Verification items for the finished model (mm, model axes). A direction names the side the tool comes from. Coordinates: 2 decimals unless noted, no trailing zeros. Order: outer loops, then holes, each group sorted by start corner. A loop starts at its lowest first (then second) coordinate and runs counter-clockwise, first axis right, second up. Notation, with made-up numbers: (-14, 42) -> (-1, 42) arc R20 ccw to (-1, 59) -> close; hole circle Ø3 at (30, 79). An arc over 180 degrees is marked (long way). Answer as CSV lines item,"result".
```python
from build123d import *

# Parameters (mm, degrees)
BOSS_EXTRUDE1_DEPTH  = 3.5
SKETCH3_R            = 4
CUT_EXTRUDE1_DEPTH   = 12.35
M5_CLEARANCE_HOLE1_D = 5.3


with BuildPart() as part:
    # Sketch1 → Boss-Extrude1 (new body)
    with BuildSketch(Plane(origin=(0, 0, 0), x_dir=(1, 0, 0), z_dir=(0, 1, 0))):
        with BuildLine():
            Line((-23.15, 0), (0, 0))
            Line((0, 0), (0, 13.4))
            ThreePointArc((0, 13.4), (-3.214400781, 13.008751962), (-6.24109589, 11.857854869))
            Line((-6.24109589, 11.857854869), (-20.532191781, 4.336081258))
            ThreePointArc((-20.532191781, 4.336081258), (-22.44480272, 2.532514588), (-23.15, 0))
        make_face()
    extrude(amount=BOSS_EXTRUDE1_DEPTH)

    # Mirror3: part across plane


with BuildPart() as part_1:
    add(part.part)
    add(part.part.mirror(Plane(origin=(0, 3.5, 0), x_dir=(0, 0, 1), z_dir=(-1, 0, 0))))

    # Mirror4: part across plane


with BuildPart() as part_2:
    add(part_1.part)
    add(part_1.part.mirror(Plane(origin=(-23.15, 3.5, 0), x_dir=(1, 0, 0), z_dir=(0, 0, -1))))

    # Sketch2 → Revolve1 (revolve)
    with BuildSketch(Plane.XY):
        Polygon((0, 0), (0, 11.35), (5.44999985, 11.35), (5.44999985, 7.99999976), (12.582539385, 7.99999976), (13.4, 3.5), (13.4, 0), align=None)
    revolve(axis=Axis((0, 0, 0), (0, 1, 0)))

    # Sketch3 → Cut-Extrude1 (cut, through all)
    with BuildSketch(Plane.XZ):
        Circle(SKETCH3_R)
    extrude(amount=-CUT_EXTRUDE1_DEPTH, mode=Mode.SUBTRACT)

    # M5 Clearance Hole1 (through all)
    with Locations(Plane(origin=(0, 0, 0), x_dir=(-1, 0, 0), z_dir=(0, -1, 0))):
        with Locations((18.25, 0), (-18.25, 0)):
            Hole(M5_CLEARANCE_HOLE1_D / 2)


solid = part_2.part
```
Item 1: Tool access check on faces 1 (the flat face through (-5, 8, 3)), 2 (the flat face through (13.29, 1.73, 8.15)). Record the directions out of +Z, -Z, +X, -X, +Y, -Y that give a thin tool (end or side, any length) a straight path to the whole face; none if there is none.
Answer list:
face 1,"+Y"
face 2,"+Z, +X, +Y, -Y"
Item 2: Section check A-A, the plane y = 2.75. Record the boundary of the cut face in (x, z), plus the area to 3 significant figures.
Answer list:
outline,"(-20.53, -4.34) -> (-6.24, -11.86) arc R13.4 ccw to (6.24, -11.86) -> (20.53, -4.34) arc R4.9 ccw to (20.53, 4.34) -> (6.24, 11.86) arc R13.4 ccw to (-6.24, 11.86) -> (-20.53, 4.34) arc R4.9 ccw to start; hole circle Ø5.3 at (-18.25, 0); hole circle Ø8 at (0, 0); hole circle Ø5.3 at (18.25, 0)"
area,"723 mm2"
Item 3: Section check D-D, the plane y = 9.5. Record the boundary of the cut face in (x, z).
Answer list:
outline,"circle Ø10.9 at (0, 0); hole circle Ø8 at (0, 0)"
Item 4: Section check B-B, the plane x = 18.25. Record the boundary of the cut face in (y, z), plus the area to 3 significant figures.
Answer list:
outline,"(0, -5.54) -> (3.5, -5.54) -> (3.5, -2.65) -> (0, -2.65) -> close; (0, 2.65) -> (3.5, 2.65) -> (3.5, 5.54) -> (0, 5.54) -> close"
area,"20.2 mm2"
Item 5: Release check for a two-part mould opening along Z. For faces 3 (the cylindrical face through (-15.722, 1.775, -0.796)), 4 (the flat face through (15, 3.5, 0)), 5 (the flat face through (-13.29, 1.73, -8.15)), 6 (the cylindrical face through (-0.867, 5.596, -3.905)) record: +Z half, -Z half, draft (parallel to the pull), parting line (faces both ways), or undercut.
Answer list:
face 3,"undercut"
face 4,"draft"
face 5,"-Z half"
face 6,"undercut"
Item 6: Thickness scan on line 1 (Y direction, x = -0.5, z = 9); line 2 (Z direction, x = 0, y = 2.5); line 3 (X direction, y = 9.75, z = -1.5). Record the ranges inside material, lowest first.
Answer list:
line 1,"0 to 8"
line 2,"-13.4 to -4, 4 to 13.4"
line 3,"-5.24 to -3.71, 3.71 to 5.24"
Item 7: Section check C-C, the plane z = -2. Count the separate pieces of the cut face and the enclosed holes in it, plus the area to 3 significant figures.
Answer list:
separate pieces,"4"
enclosed holes,"0"
area,"206 mm2"
Item 8: Depth check by flat-ended pin: pin 1 Ø5 at (x, z) = (-13, -5) entering from +Y; pin 2 Ø2 at (y, z) = (6, -2) entering from -X; pin 3 Ø6 at (x, y) = (-7, 8.5) entering from +Z. Enter the tip coordinate at first touch or a pass-through.
Answer list:
pin 1,"y = 8"
pin 2,"x = -13.02"
pin 3,"z = 11.98"
